Job drawing, mm, ordinate dimensions from the low corner. One solid piece. Coordinates: 2 decimals unless noted, no trailing zeros. Order: outer loops, then holes, each group sorted by start corner. A loop starts at its lowest first (then second) coordinate and runs counter-clockwise, first axis right, second up. Notation, with made-up numbers: M -27,32.5 L -19,32.5 A21 cw -19,50.5 Z; hole C -26,2 d3. An arc over 180 degrees is marked long. Write item = value, one per line.
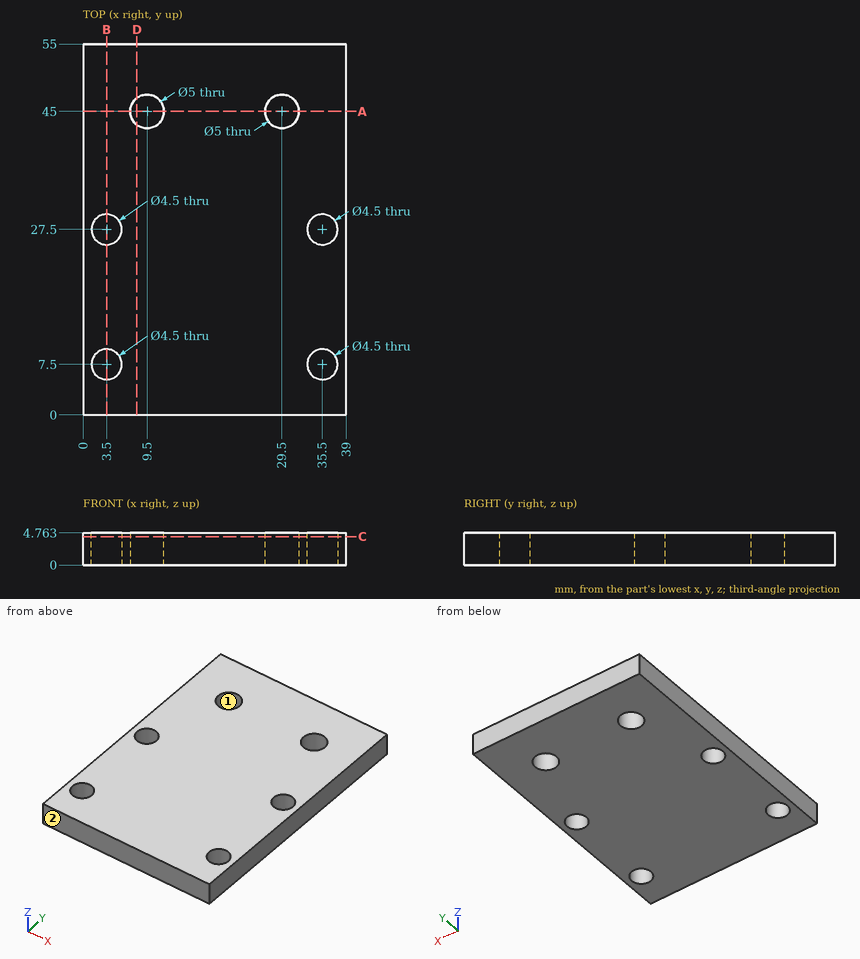
(1) Slice it at C-C, the plane z = 4.2. Write the cut outline in (x, y), then the cut area to 3 significant figures.
Evaluation:
outline = M 0,0 L 39,0 L 39,55 L 0,55 Z; hole C 3.5,7.5 d4.5; hole C 3.5,27.5 d4.5; hole C 9.5,45 d5; hole C 29.5,45 d5; hole C 35.5,7.5 d4.5; hole C 35.5,27.5 d4.5
area = 2,040 mm²
(2) Slice it at B-B, the plane x = 3.5. Write the cut outline in (y, z).
Evaluation:
outline = M 0,0 L 5.25,0 L 5.25,4.76 L 0,4.76 Z; M 9.75,0 L 25.25,0 L 25.25,4.76 L 9.75,4.76 Z; M 29.75,0 L 55,0 L 55,4.76 L 29.75,4.76 Z
(3) Pull direction X, two halves, no side cores. Call the marked faces 1 and 2: +X half, -X half, draft (parallel to the pull), parting line (faces both ways), or undercut.
Evaluation:
face_1 = undercut
face_2 = draft
(4) Slice it at A-A, the plane y = 45. Write the cut outline in (x, z).
Evaluation:
outline = M 0,0 L 7,0 L 7,4.76 L 0,4.76 Z; M 12,0 L 27,0 L 27,4.76 L 12,4.76 Z; M 32,0 L 39,0 L 39,4.76 L 32,4.76 Z
(5) Wall check: line 1 (X direction, y = 7.5, z = 3.75); line 2 (Y direction, x = 3.5, z = 3.1); line 3 (X direction, y = 45, z = 2.5). Give the ranges that are in metal, low to high. Write a range as from..to.
Evaluation:
line_1 = 0..1.25, 5.75..33.25, 37.75..39
line_2 = 0..5.25, 9.75..25.25, 29.75..55
line_3 = 0..7, 12..27, 32..39
(6) Slice it at D-D, the plane x = 8. Write the cut outline in (y, z), then the cut area to 3 significant figures.
Evaluation:
outline = M 0,0 L 43,0 L 43,4.76 L 0,4.76 Z; M 47,0 L 55,0 L 55,4.76 L 47,4.76 Z
area = 243 mm²
(7) Pin check, flat tips, straight feed: pin 1 Ø12 at (x, y) = (13.5, 12) entering from -Z; pin 2 Ø3 at (x, y) = (9.5, 45) entering from +Z. Stop position of each tip, or through.
Evaluation:
pin_1 = 0
pin_2 = through
